from build123d import *

# Parameters (mm, degrees)
F0_W        = 36.83
F0_H        = 2.54
F1_DEPTH    = 12.7
F3_T1_DEPTH = 58.8270452561
F4_DEPTH    = 25.4


# Not quite as in the source:
# - a fillet or chamfer that OpenCascade refuses, or shapes differently, is made with other operations: its cross-section is extruded or revolved along the edge and cut away or added


with BuildPart() as f1:
    # F0 (on Top) → F1 (new body)
    with BuildSketch(Plane.XY):
        with Locations((-0.635, 1.27)):
            Rectangle(F0_W, F0_H)
    extrude(amount=F1_DEPTH)

    # F3: fillet of radius 5.08 on 1 edges, made by hand

    # F3_s2 → F3_t1 (cut)
    with BuildSketch(Plane.YZ.offset(-30.0485226281)):
        with BuildLine():
            ThreePointArc((2.54, 8.3005909488), (1.8594090512, 10.8405909488), (0, 12.7))
            Line((0, 12.7), (2.54, 12.7))
            Line((2.54, 12.7), (2.54, 8.3005909488))
        make_face()
    extrude(amount=F3_T1_DEPTH, mode=Mode.SUBTRACT)

    # F2 (on face) → F4 (cut)
    with BuildSketch(Plane.XZ):
        Polygon((-15.875, 11.2622954744), (-15.0449409051, 12.7), (-16.7050590949, 12.7), align=None)
        Polygon((-4.7382939367, 12.7), (-6.6917060633, 12.7), (-5.715, 11.0082954744), align=None)
        Polygon((5.2750590949, 12.7), (3.6149409051, 12.7), (4.445, 11.2622954744), align=None)
        Polygon((15.4350590949, 12.7), (13.7749409051, 12.7), (14.605, 11.2622954744), align=None)
    extrude(amount=-F4_DEPTH, mode=Mode.SUBTRACT)


solid = f1.part
Input: part model. Units: mm. Frame: model coordinates. Give positions to 0.01 mm unless a question says otherwise; leave off trailing zeros. Order: outer loops, then holes, each group sorted by start corner. A loop starts at its lowest first (then second) coordinate and runs counter-clockwise, first axis right, second up. Notation, with made-up numbers: (35, 69) - (59, 69) arc R21 cw to (59, 92) - close; hole circle Ø7 at (55, 12.5). An arc over 180 degrees is marked (long way). Answer as a JSON object with one key per item and string values. Group by question number.
Q1. Cut plane C-C, the plane z = 9. Output: boundary loops of the cut face in (x, y).
Q2. Mould query, pull axis X, two halves, no side actions, for faces 1 (the face through (-1, 2.54, 4)), 2 (the face through (-16.204, 0.606, 11.831)), 3 (the face through (17.78, 1, 6)). Classes: pulls with the +X half, pulls with the -X half, needs draft (parallel to the pull), parting line crosses it, or undercut.
Q3. Cut plane A-A, the plane x = -7.5. Output: boundary loops of the cut face in (y, z), then the cut area to 3 significant figures.
Q4. Cut plane B-B, the plane y = 0.55. Output: boundary loops of the cut face in (x, z) (3 decimals), then the cut area to 3 significant figures.
Q5. Line query: probe 1 along X at (y, z) = (1.05, 11.5); probe 2 along Y at (x, z) = (-12, 11.25); probe 3 along Z at (x, y) = (-5.5, 1.75). Output: solid intervals per line, ascending.
Q6. Cut plane D-D, the plane x = -15.5. Output: boundary loops of the cut face in (y, z).
Results:
{
 "1": {"outline": "(-19.05, 0) - (17.78, 0) - (17.78, 2.49) - (-19.05, 2.49) - close"},
 "2": {"face 1": "needs draft", "face 2": "undercut", "face 3": "pulls with the +X half"},
 "3": {"outline": "(0, 0) - (2.54, 0) - (2.54, 8.3) arc R5.08 ccw to (0, 12.7) - close", "area": "29.0 mm^2"},
 "4": {"outline": "(-19.05, 0) - (17.78, 0) - (17.78, 12.333) - (15.223, 12.333) - (14.605, 11.262) - (13.987, 12.333) - (5.063, 12.333) - (4.445, 11.262) - (3.827, 12.333) - (-4.95, 12.333) - (-5.715, 11.008) - (-6.48, 12.333) - (-15.257, 12.333) - (-15.875, 11.262) - (-16.493, 12.333) - (-19.05, 12.333) - close", "area": "451 mm^2"},
 "5": {"probe 1": "-19.05 to -16.01, -15.74 to -6, -5.43 to 4.31, 4.58 to 14.47, 14.74 to 17.78", "probe 2": "0 to 1.6", "probe 3": "0 to 11.02"},
 "6": {"outline": "(0, 0) - (2.54, 0) - (2.54, 8.3) arc R5.08 ccw to (1.03, 11.91) - (0, 11.91) - close"}
}
